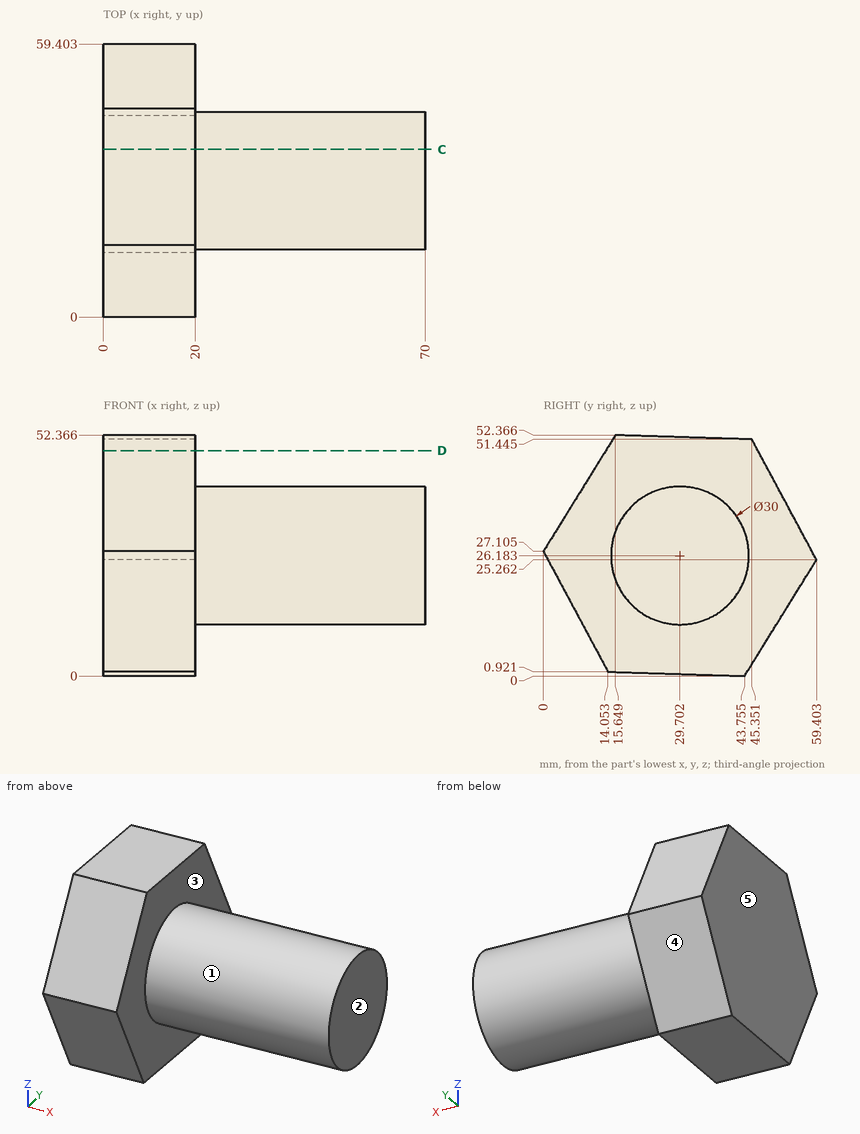
Print and shaded views of the part. All mm, measured from the part's lowest x, y and z. A direction names the side the tool comes from. Round coordinates to 2 decimals unless told otherwise and drop trailing zeros. Write each loop counter-clockwise with the first axis right and the second up, starting at its lowest first coordinate (ties: lowest second). Pieces come first, ordered by that corner, then holes.
(1) Slice it at D-D, the plane z = 49. Write the cut outline in (x, y).
(2) Probe line 1 along X through (y, z) = (40, 39.5); line 2 along Z through (x, y) = (18, 23.5); line 3 along Z through (x, y) = (31, 21) (1 decimal). List the from-to ranges inside material, lowest first.
(3) 3-axis set-ups, long thin cutter, end or side, ignore diameter. For the marked faces 1 and 2: which of +Z, -Z, +X, -X, +Y, -Y reach the whole face in a straight line?
(4) Drop flat-ended pins along their axis: P1, Ø5, axis at x = 54.5, y = 37, coming from the -Z side; P2, Ø8, axis at x = 31, y = 32.5, coming from the +Z side; P3, Ø12, axis at x = 19, y = 40.5, coming from the +Z side. Give the stop position or say it passes through.
(5) Mould opens along X. For the marked faces 3, 4 and 5 say: pulls with the +X half, pulls with the -X half, needs draft (parallel to the pull), parting line crosses it, or undercut.
(6) Slice it at C-C, the plane y = 36.5. Write the cut outline in (x, z) (1 decimal).
From the geometry:
1. outline: (0, 13.56) - (20, 13.56) - (20, 46.66) - (0, 46.66) - close
2. line 1: x = 0 to 20
2. line 2: z = 0.63 to 52.12
2. line 3: z = 14 to 38.4
3. face 1: +X
3. face 2: +Z, -Z, +X, +Y, -Y
4. P1: stops at z = 11.97
4. P2: stops at z = 41.18
4. P3: stops at z = 51.78
5. face 3: pulls with the +X half
5. face 4: needs draft
5. face 5: pulls with the -X half
6. outline: (0, 0.2) - (20, 0.2) - (20, 12.8) - (70, 12.8) - (70, 39.6) - (20, 39.6) - (20, 51.7) - (0, 51.7) - close
